Read the model definition and answer for the solid it produces. Units are mm, in the model's axes. Face numbers are marked on the shaded views. A direction names the side the tool comes from. Coordinates: 2 decimals unless noted, no trailing zeros. Loops run counter-clockwise (first coordinate to the right, second up) from the corner with the lowest first, then second, coordinate; pieces in that order, holes last. Notation, with made-up numbers: M 36.25,30.25 L 54.25,30.25 A5 cw 54.25,37.25 Z; hole C 6,69 d5. An arc over 180 degrees is marked long. One line per item, written item: value. Start each with the question number.
1. Flat-ended cylindrical pins translate along their axes: pin 1 (4.5 mm diameter, centred on x = 4.95, y = 6.65, fed in from -Z); pin 2 (5 mm diameter, centred on y = -8, z = 3.5, fed in from -X); pin 3 (2 mm diameter, centred on x = 3.5, y = -4, fed in from -Z). Find the tip coordinate at first contact, or state that the pin passes through.
2. For the marked faces 1, 2 and 3, determine the directions among +Z, -Z, +X, -X, +Y, -Y from which every point of the face is accessible in a straight line to the end or side of a thin tool.
3. The part is cut by section B-B (y = -3.7). Write down the section's boundary in (x, z).
4. The part is cut by section A-A (z = 1.5). Write down the section's boundary in (x, y).
5. Consider probe 1 along X at (y, z) = (-3.7, 3); probe 2 along X at (y, z) = (6.65, 3); probe 3 along Y at (x, z) = (-8.5, 6.25). Determine where each line is inside the solid, lowest interval first.
6. The part is cut by section D-D (z = 9). Write down the section's boundary in (x, y), then the cut area to 3 significant figures.
7. The part is cut by section C-C (x = 0). Write down the section's boundary in (y, z).
8. Determine the mould class of the marked faces 4, 5 and 6 for opening direction X: +X half, -X half, draft (parallel to the pull), parting line (faces both ways), or undercut.
```python
from build123d import *

# Parameters (mm, degrees)
F1_DEPTH     = 10.25
F3_DEPTH     = 2.25
F4_R         = 1
F5_T         = 1.9
F5_T3_DEPTH  = 4.8
F5_T5_DEPTH  = 27.8972844735
F5_T8_ANGLE  = 90.000000001
F5_T10_ANGLE = 90.000000001
F6_R         = 3.75
F6_R_2       = 2.55
F7_DEPTH     = 8
F8_R         = 3.5
F8_R_2       = 1.25
F9_DEPTH     = 8
F10_R        = 3.75
F10_R_2      = 2.55
F11_DEPTH    = 8
F13_DEPTH    = 6


# Not quite as in the source:
# - a shell that OpenCascade refuses in one call is made with other operations: the cavity is built on its own and cut out


with BuildPart() as f1:
    # F0 (on Top) → F1 (new body)
    with BuildSketch(Plane.XY):
        with BuildLine():
            Line((11, 24), (-11, 24))
            ThreePointArc((-11, 24), (-16.6568542495, 21.6568542495), (-19, 16))
            Line((-19, 16), (-19, -16))
            ThreePointArc((-19, -16), (-16.6568542495, -21.6568542495), (-11, -24))
            Line((-11, -24), (11, -24))
            ThreePointArc((11, -24), (16.6568542495, -21.6568542495), (19, -16))
            Line((19, -16), (19, 16))
            ThreePointArc((19, 16), (16.6568542495, 21.6568542495), (11, 24))
        make_face()
    extrude(amount=F1_DEPTH)

    # F2 (on face) → F3 (join)
    with BuildSketch(Plane.XY.offset(10.25)):
        with BuildLine():
            ThreePointArc((-19, 16), (-16.6568542495, 21.6568542495), (-11, 24))
            Line((-11, 24), (-11.85, 24))
            ThreePointArc((-11.85, 24), (-18.9210678119, 21.0710678119), (-21.85, 14))
            Line((-21.85, 14), (-21.85, -8.0972844735))
            Line((-21.85, -8.0972844735), (-19, -8.0972844735))
            Line((-19, -8.0972844735), (-19, 16))
        make_face()
        with BuildLine():
            Line((21.85, -5.7972865179), (21.85, 14))
            ThreePointArc((21.85, 14), (18.9210678119, 21.0710678119), (11.85, 24))
            Line((11.85, 24), (11, 24))
            ThreePointArc((11, 24), (16.6568542495, 21.6568542495), (19, 16))
            Line((19, 16), (19, -8.0972844735))
            Line((19, -8.0972844735), (21.85, -8.0972844735))
            Line((21.85, -8.0972844735), (21.85, -5.7972865179))
        make_face()
    extrude(amount=-F3_DEPTH)

    # F4
    f4_edges = [f1.edges().sort_by_distance(p)[0] for p in [
        (21.85, -8.097284, 9.125),
        (19, -8.097284, 9.125),
        (-21.85, -8.097284, 9.125),
        (-19, -8.097284, 9.125),
    ]]
    fillet(f4_edges, radius=F4_R)

    # F5: shell of thickness 1.9, made by hand


with BuildPart() as f5_core1:
    # F5_t2: copy of F1
    add(f1.part)

    # the walls: a layer under each face that stays
    f5_faces = [f5_core1.faces().sort_by_distance(p)[0] for p in [
        (19, 0, 5.125),
        (0, 0, 10.25),
        (19.2928932188, -8.3901776923, 9.125),
        (16.6568542495, -21.6568542495, 5.125),
        (20.0416666667, -3.5810703946, 8),
        (16.6568542495, 21.6568542495, 4),
        (-21.85, 3.4513577633, 9.125),
        (-18.9210678119, 21.0710678119, 9.125),
        (-20.425, -8.0972844735, 9.125),
        (0, 24, 5.125),
        (-19.2928932188, -8.3901776923, 9.125),
        (18.9210678119, 21.0710678119, 9.125),
        (-19, 0, 5.125),
        (21.85, 3.4513577633, 9.125),
        (-16.6568542495, -21.6568542495, 5.125),
        (0, -24, 5.125),
        (20.425, -8.0972844735, 9.125),
        (-16.6568542495, 21.6568542495, 4),
        (-20.0416666667, -3.5810703946, 8),
    ]]
    thicken(f5_faces, amount=-F5_T, mode=Mode.SUBTRACT)

    # F5_s4 → F5_t3 (cut)
    with BuildSketch(Plane.XZ.offset(6.1972844735)):
        Polygon((19.019, 7.981), (17.1, 8), (17.1, 9.9), (19, 9.9), align=None)
        Polygon((-19.019, 7.981), (-17.1, 8), (-17.1, 9.9), (-19, 9.9), align=None)
    extrude(amount=F5_T3_DEPTH, mode=Mode.SUBTRACT)

    # F5_s6 → F5_t5 (cut)
    with BuildSketch(Plane.XZ.offset(-17.9)):
        Polygon((19.019, 7.981), (17.1, 8), (17.1, 9.9), (19, 9.9), align=None)
        Polygon((-19.019, 7.981), (-17.1, 8), (-17.1, 9.9), (-19, 9.9), align=None)
    extrude(amount=F5_T5_DEPTH, mode=Mode.SUBTRACT)

    # F5_s7 → F5_t8 (revolve, cut)
    with BuildSketch(Plane.YZ.offset(11)):
        Polygon((24.019, 7.981), (24, 9.9), (22.1, 9.9), (22.1, 8), align=None)
    revolve(axis=Axis((11, 16, 8), (0, 0, -1)), revolution_arc=F5_T8_ANGLE, mode=Mode.SUBTRACT)

    # F5_s9 → F5_t10 (revolve, cut)
    with BuildSketch(Plane.XZ.offset(-16)):
        Polygon((-19.019, 7.981), (-17.1, 8), (-17.1, 9.9), (-19, 9.9), align=None)
    revolve(axis=Axis((-11, 16, 8), (0, 0, -1)), revolution_arc=F5_T10_ANGLE, mode=Mode.SUBTRACT)


with BuildPart() as f1_1:
    add(f1.part)

    # what is left inside the walls is the cavity
    f5_cavity = [f5_core1.part.solids().sort_by_distance(p)[0] for p in [
        (0, -7.366667, 0.019),
    ]]
    add(f5_cavity, mode=Mode.SUBTRACT)

    # F6 (on face) → F7 (join)
    with BuildSketch(Plane(origin=(0, 0, 8.35), x_dir=(1, 0, 0), z_dir=(0, 0, -1))):
        with Locations((1.35, 16.1)):
            Circle(F6_R)
        with Locations((1.35, 16.1)):
            Circle(F6_R_2, mode=Mode.SUBTRACT)
    extrude(amount=F7_DEPTH)

    # F8 (on face) → F9 (join)
    with BuildSketch(Plane(origin=(0, 0, 8.35), x_dir=(1, 0, 0), z_dir=(0, 0, -1))):
        with Locations((1.8068233039, 3.7)):
            Circle(F8_R)
        with Locations((1.8068233039, 3.7)):
            Circle(F8_R_2, mode=Mode.SUBTRACT)
    extrude(amount=F9_DEPTH)

    # F10 (on face) → F11 (join)
    with BuildSketch(Plane(origin=(0, 0, 8.35), x_dir=(1, 0, 0), z_dir=(0, 0, -1))):
        with Locations((4.9459114671, -6.65)):
            Circle(F10_R)
        with Locations((4.9459114671, -6.65)):
            Circle(F10_R_2, mode=Mode.SUBTRACT)
    extrude(amount=F11_DEPTH)

    # F12 (on face) → F13 (join)
    with BuildSketch(Plane(origin=(0, 0, 8.35), x_dir=(1, 0, 0), z_dir=(0, 0, -1))):
        with BuildLine():
            ThreePointArc((1.9864868995, 12.4044101382), (1.4880585521, 12.3525422169), (0.987164824, 12.3675945243))
            Line((0.987164824, 12.3675945243), (1.1796292386, 7.1433454088))
            ThreePointArc((1.1796292386, 7.1433454088), (1.6779686553, 7.1976272642), (2.1789513141, 7.1801610227))
            Line((2.1789513141, 7.1801610227), (1.9864868995, 12.4044101382))
        make_face()
    extrude(amount=F13_DEPTH)


solid = f1_1.part
```
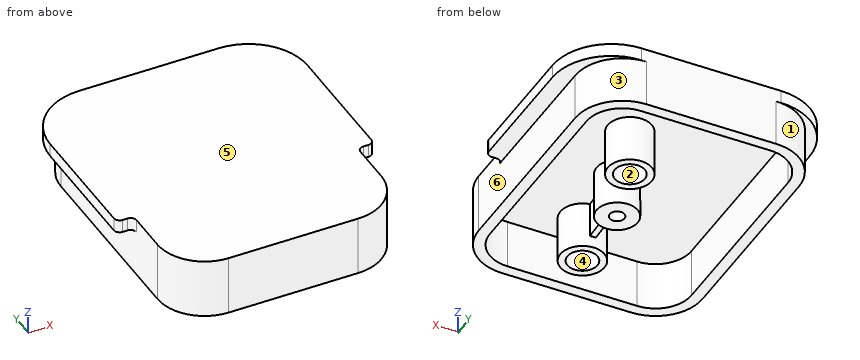
Answer block:
1. pin 1: stops at z = 8.35
1. pin 2: stops at x = -19
1. pin 3: stops at z = 0.35
2. face 1: -Z, -X, +Y
2. face 2: -Z
2. face 3: -Z, +X, +Y
3. outline: M -21.85,8 L -19,8 L -19,0 L -17.1,0 L -17.1,8.35 L -1.69,8.35 L -1.69,0.35 L 0.56,0.35 L 0.56,8.35 L 3.06,8.35 L 3.06,0.35 L 5.31,0.35 L 5.31,8.35 L 17.1,8.35 L 17.1,0 L 19,0 L 19,8 L 21.85,8 L 21.85,10.25 L -21.85,10.25 Z
4. outline: M -19,-16 A8 ccw -11,-24 L 11,-24 A8 ccw 19,-16 L 19,16 A8 ccw 11,24 L -11,24 A8 ccw -19,16 Z; C 1.35,-16.1 d7.5; C 1.81,-3.7 d7; C 4.95,6.65 d7.5; hole M -17.1,-16 A6.1 ccw -11,-22.1 L 11,-22.1 A6.1 ccw 17.1,-16 L 17.1,16 A6.1 ccw 11,22.1 L -11,22.1 A6.1 ccw -17.1,16 Z; hole C 1.35,-16.1 d5.1; hole C 1.81,-3.7 d2.5; hole C 4.95,6.65 d5.1
5. probe 1: x = -19 to -17.1, -1.69 to 0.56, 3.06 to 5.31, 17.1 to 19
5. probe 2: x = -19 to -17.1, 1.2 to 2.4, 7.5 to 8.7, 17.1 to 19
5. probe 3: y = -24 to -22.1, 22.1 to 24
6. outline: M -21.85,-7.1 A1 ccw -20.85,-8.1 L -20,-8.1 A1 cw -19,-9.1 L -19,-16 A8 ccw -11,-24 L 11,-24 A8 ccw 19,-16 L 19,-9.1 A1 cw 20,-8.1 L 20.85,-8.1 A1 ccw 21.85,-7.1 L 21.85,14 A10 ccw 11.85,24 L -11.85,24 A10 ccw -21.85,14 Z
6. area: 1,940 mm2
7. outline: M -24,0 L -22.1,0 L -22.1,8.35 L -19.6,8.35 L -19.6,0.35 L -18.26,0.35 L -18.26,8.35 L -13.94,8.35 L -13.94,0.35 L -12.6,0.35 L -12.6,8.35 L -6.7,8.35 L -6.7,0.35 L -0.7,0.35 L -0.7,8.35 L 22.1,8.35 L 22.1,0 L 24,0 L 24,10.25 L -24,10.25 Z
8. face 4: undercut
8. face 5: draft
8. face 6: +X half
